Geometry check sheet. Reference: drawing and pictorial views, mm from the part's lowest x, y, z. Coordinates: 2 decimals unless noted, no trailing zeros. Loops run counter-clockwise (first coordinate to the right, second up) from the corner with the lowest first, then second, coordinate; pieces in that order, holes last.
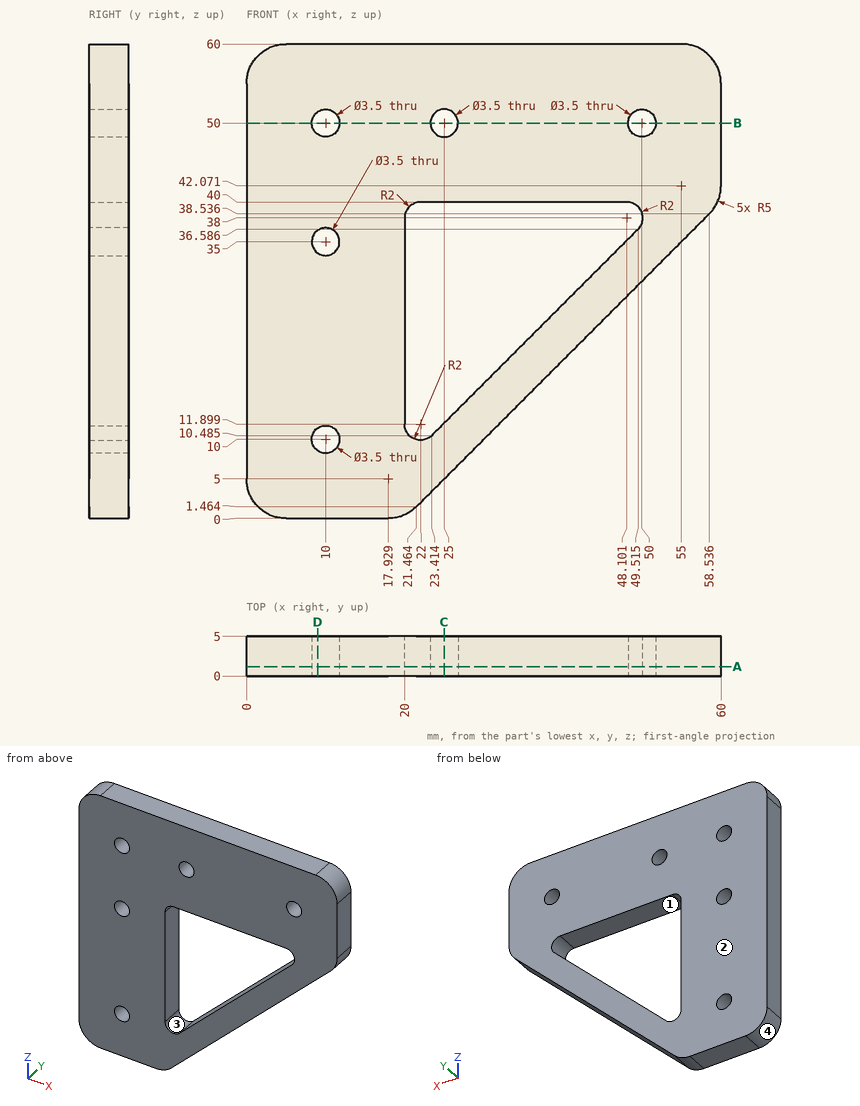
1) Section check C-C on x = 25. Record the cut outline in (y, z), and give its area (3 significant figures).
Data:
outline: (0, 5) - (5, 5) - (5, 12.07) - (0, 12.07) - close; (0, 40) - (5, 40) - (5, 48.25) - (0, 48.25) - close; (0, 51.75) - (5, 51.75) - (5, 60) - (0, 60) - close
area: 118 mm2
2) Depth check by flat-ended pin: pin 1 (5 mm diameter, centred on x = 26.5, z = 20, fed in from +Y); pin 2 (3 mm diameter, centred on y = 2, z = 13, fed in from +X); pin 3 (3 mm diameter, centred on x = 45, y = 0.5, fed in from -Z). Enter the tip coordinate at first touch or a pass-through.
Data:
pin 1: passes through
pin 2: stops at x = 34.5
pin 3: stops at z = 23.5
3) Section check D-D on x = 9. Record the cut outline in (y, z).
Data:
outline: (0, 0) - (5, 0) - (5, 8.56) - (0, 8.56) - close; (0, 11.44) - (5, 11.44) - (5, 33.56) - (0, 33.56) - close; (0, 36.44) - (5, 36.44) - (5, 48.56) - (0, 48.56) - close; (0, 51.44) - (5, 51.44) - (5, 60) - (0, 60) - close
4) Material ranges on probe 1 along X at (y, z) = (3, 50); probe 2 along X at (y, z) = (3.5, 38); probe 3 along X at (y, z) = (2.35, 39) (1 decimal), recorded low to high.
Data:
probe 1: x = 0 to 8.25, 11.75 to 23.25, 26.75 to 48.25, 51.75 to 60
probe 2: x = 0 to 20, 50.1 to 58
probe 3: x = 0 to 20.3, 49.8 to 58.9
5) Section check A-A on y = 1.2. Count the separate pieces of the cut face and the enclosed holes in it, and give its area (3 significant figures).
Data:
separate pieces: 1
enclosed holes: 6
area: 2,200 mm2
6) Section check B-B on z = 50. Record the cut outline in (x, y).
Data:
outline: (0, 0) - (8.25, 0) - (8.25, 5) - (0, 5) - close; (11.75, 0) - (23.25, 0) - (23.25, 5) - (11.75, 5) - close; (26.75, 0) - (48.25, 0) - (48.25, 5) - (26.75, 5) - close; (51.75, 0) - (60, 0) - (60, 5) - (51.75, 5) - close
7) Mould release check, pull along X, two halves, no side actions. Record for the marked faces 1, 2, 3 and 4: +X half, -X half, draft (parallel to the pull), parting line (faces both ways), or undercut.
Data:
face 1: undercut
face 2: draft
face 3: undercut
face 4: -X half
